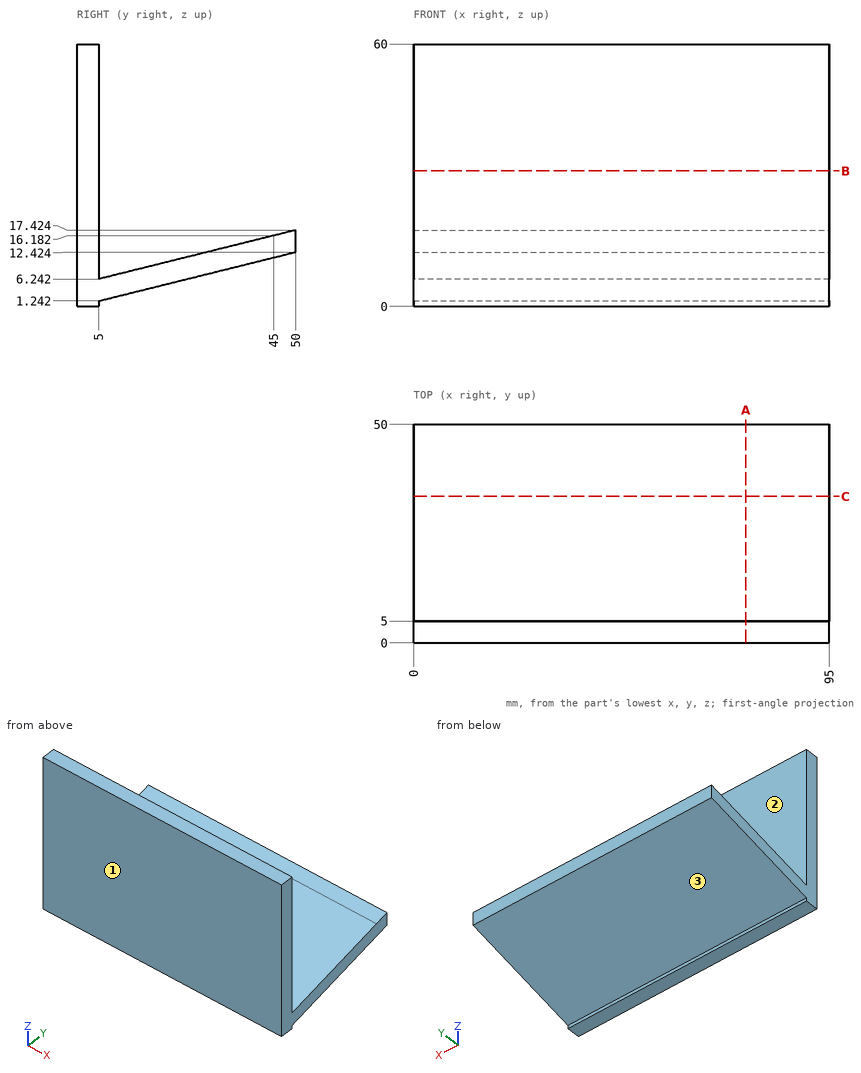
Can you work these out from the drawing? Everything is in mm from the part's minimum corner. Coordinates: 2 decimals unless noted, no trailing zeros. Write each loop counter-clockwise with the first axis right and the second up, starting at its lowest first coordinate (ties: lowest second). Pieces come first, ordered by that corner, then holes. Notation, with made-up numbers: (87.5, 44.25) - (95.5, 44.25) arc R13 ccw to (95.5, 50.25) - close; hole circle Ø3 at (86.25, 19.25). An arc over 180 degrees is marked (long way). One line per item, written item: value.
1) Suppose I cut it at A-A on x = 76. Write out the boundary of the cut face in (y, z) (1 decimal), and give its area (3 significant figures).
Model answer:
outline: (0, 0) - (5, 0) - (5, 1.2) - (50, 12.4) - (50, 17.4) - (5, 6.2) - (5, 60) - (0, 60) - close
area: 525 mm²
2) We'd pull the mould along Y, two halves only. Please class the marked faces 1, 2 and 3: pulls with the +Y half, pulls with the -Y half, needs draft (parallel to the pull), parting line crosses it, or undercut.
Model answer:
face 1: pulls with the -Y half
face 2: undercut
face 3: pulls with the +Y half
3) Suppose I cut it at C-C on y = 33.5. Write out the boundary of the cut face in (x, z) (1 decimal), and give its area (3 significant figures).
Model answer:
outline: (0, 8.3) - (95, 8.3) - (95, 13.3) - (0, 13.3) - close
area: 475 mm²
4) Suppose I cut it at B-B on z = 31. Write out the boundary of the cut face in (x, y).
Model answer:
outline: (0, 0) - (95, 0) - (95, 5) - (0, 5) - close
5) I'm going to push flat-ended pins straight in: P1, Ø8, axis at x = 52, z = 23, coming from the +Y side; P2, Ø2, axis at x = 18.5, y = 43, coming from the +Z side; P3, Ø3, axis at x = 52.5, y = 16.5, coming from the +Z side. Where does each tip first touch, or does it pass through?
Model answer:
P1: stops at y = 5
P2: stops at z = 15.93
P3: stops at z = 9.47
6) I need wall thicknesses on line 1 along Y through (x, z) = (47.5, 56.5); line 2 along Z through (x, y) = (27, 18); line 3 along Z through (x, y) = (89, 46). Which ranges of each line are inside material? Lowest first, please.
Model answer:
line 1: y = 0 to 5
line 2: z = 4.47 to 9.47
line 3: z = 11.43 to 16.43
